Can you work these out from the model? Positions are in its coordinate system, mm. A direction names the side the tool comes from. Coordinates: 2 decimals unless noted, no trailing zeros. Loops run counter-clockwise (first coordinate to the right, second up) from the corner with the lowest first, then second, coordinate; pieces in that order, holes last.
```python
from build123d import *

# Parameters (mm, degrees)
BOSS_EXTRUDE1_DEPTH     = 46
BOSS_EXTRUDE2_DEPTH     = 54
CUT_EXTRUDE1_DEPTH      = 133.4990566
CUT_EXTRUDE1_DEPTH_BACK = 133.4990566
CUT_EXTRUDE2_DEPTH      = 126.888839855
CUT_EXTRUDE2_DEPTH_BACK = 126.888839855
F_12_0MM_DOWEL_HOLE1_D  = 12
SKETCH14_W              = 28
SKETCH14_H              = 28
SKETCH14_R              = 6
CUT_EXTRUDE5_DEPTH      = 10
SKETCH15_R              = 4
CUT_EXTRUDE6_DEPTH      = 54
CUT_EXTRUDE7_DEPTH      = 21
CHAMFER2_SIZE           = 2
FILLET1_R               = 8
CHAMFER3_SIZE           = 1


with BuildPart() as part:
    # Sketch1 → Boss-Extrude1 (new body)
    with BuildSketch(Plane.XY):
        Polygon((-104, 0), (104, 0), (99.985564599, 14), (-99.985564599, 14), align=None)
    extrude(amount=BOSS_EXTRUDE1_DEPTH)

    # Sketch2 → Boss-Extrude2 (add)
    with BuildSketch(Plane(origin=(0, 14, 0), x_dir=(1, 0, 0), z_dir=(0, 1, 0))):
        with BuildLine():
            Line((-48.856934001, 0), (48.856934001, 0))
            ThreePointArc((48.856934001, 0), (54, -23), (48.856934001, -46))
            Line((48.856934001, -46), (-48.856934001, -46))
            ThreePointArc((-48.856934001, -46), (-54, -23), (-48.856934001, 0))
        make_face()
    extrude(amount=BOSS_EXTRUDE2_DEPTH)

    # Sketch3 → Cut-Extrude1 (cut, two sides: drawn at the far end of the back side and taken through both)
    with BuildSketch(Plane.XY.offset(46).offset(-CUT_EXTRUDE1_DEPTH_BACK)):
        with BuildLine():
            Line((28, 52), (28, 68))
            Line((28, 68), (-28, 68))
            Line((-28, 68), (-28, 52))
            Line((-28, 52), (-23.664319132, 52))
            ThreePointArc((-23.664319132, 52), (0, 24), (23.664319132, 52))
            Line((23.664319132, 52), (28, 52))
        make_face()
    extrude(amount=CUT_EXTRUDE1_DEPTH + CUT_EXTRUDE1_DEPTH_BACK, mode=Mode.SUBTRACT)

    # Sketch4 → Cut-Extrude2 (cut, two sides: drawn at the far end of the back side and taken through both)
    with BuildSketch(Plane(origin=(0, 14, 0), x_dir=(1, 0, 0), z_dir=(0, 1, 0)).offset(-CUT_EXTRUDE2_DEPTH_BACK)):
        with BuildLine():
            Line((77, -17), (85, -17))
            ThreePointArc((85, -17), (91, -23), (85, -29))
            Line((85, -29), (77, -29))
            ThreePointArc((77, -29), (71, -23), (77, -17))
        make_face()
        with BuildLine():
            Line((-77, -17), (-85, -17))
            ThreePointArc((-85, -17), (-91, -23), (-85, -29))
            Line((-85, -29), (-77, -29))
            ThreePointArc((-77, -29), (-71, -23), (-77, -17))
        make_face()
    extrude(amount=CUT_EXTRUDE2_DEPTH + CUT_EXTRUDE2_DEPTH_BACK, mode=Mode.SUBTRACT)

    # Ø12.0mm Dowel Hole1 (through all)
    with Locations(Plane(origin=(0, 68, 0), x_dir=(1, 0, 0), z_dir=(0, 1, 0))):
        with Locations((39, -23)):
            f_12_0mm_dowel_hole1 = Hole(F_12_0MM_DOWEL_HOLE1_D / 2)

    # Mirror1: Ø12.0mm Dowel Hole1 across plane
    add(f_12_0mm_dowel_hole1.mirror(Plane(origin=(0, 0, 0), x_dir=(0, 0, 1), z_dir=(1, 0, 0))), mode=Mode.SUBTRACT)

    # Sketch14 → Cut-Extrude5 (cut)
    # profile 1 of 2: a face of its own
    with BuildSketch(Plane.XZ):
        with Locations((-39, 23)):
            Rectangle(SKETCH14_W, SKETCH14_H)
        with Locations(Location((-39, 23, 0), (0, 0, 90))):
            Circle(SKETCH14_R, mode=Mode.SUBTRACT)
    # profile 2 of 2: a face of its own
    with BuildSketch(Plane.XZ):
        with Locations((39, 23)):
            Rectangle(SKETCH14_W, SKETCH14_H)
        with Locations(Location((39, 23, 0), (0, 0, 90))):
            Circle(SKETCH14_R, mode=Mode.SUBTRACT)
    extrude(amount=-CUT_EXTRUDE5_DEPTH, mode=Mode.SUBTRACT)

    # Sketch15 → Cut-Extrude6 (cut)
    with BuildSketch(Plane(origin=(0, 68, 0), x_dir=(1, 0, 0), z_dir=(0, 1, 0))):
        with Locations(Location((0, -23, 0), (0, 0, 180))):
            Circle(SKETCH15_R)
    extrude(amount=-CUT_EXTRUDE6_DEPTH, mode=Mode.SUBTRACT)

    # Sketch18 → Cut-Extrude7 (cut, symmetric)
    with BuildSketch(Plane.XY.offset(23)):
        Polygon((-97.5, 0), (-96.926509228, 2), (96.926509228, 2), (97.5, 0), align=None)
    extrude(amount=CUT_EXTRUDE7_DEPTH, both=True, mode=Mode.SUBTRACT)

    # Chamfer2
    chamfer2_edges = [part.edges().sort_by_distance(p)[0] for p in [
        (0, 24, 0),
        (0, 24, 46),
    ]]
    chamfer(chamfer2_edges, length=CHAMFER2_SIZE)

    # Fillet1
    fillet1_edges = [part.edges().sort_by_distance(p)[0] for p in [
        (54, 14, 23),
        (-54, 14, 23),
    ]]
    fillet(fillet1_edges, radius=FILLET1_R)

    # Chamfer3
    chamfer3_edges = [part.edges().sort_by_distance(p)[0] for p in [
        (-71, 14, 23),
        (-81, 14, 29),
        (-91, 14, 23),
        (-81, 14, 17),
        (81, 14, 17),
        (81, 14, 29),
        (91, 14, 23),
        (71, 14, 23),
    ]]
    chamfer(chamfer3_edges, length=CHAMFER3_SIZE)


solid = part.part
```
(1) I want a section at D-D on x = -38. Write out the boundary of the cut face in (y, z), then the cut area to 3 significant figures.
Check values:
outline: (0, 0) - (68, 0) - (68, 17.08) - (10, 17.08) - (10, 9) - (2, 9) - (2, 2) - (0, 2) - close; (0, 44) - (2, 44) - (2, 37) - (10, 37) - (10, 28.92) - (68, 28.92) - (68, 46) - (0, 46) - close
area: 2,130 mm2
(2) I want a section at B-B on x = 39. Write out the boundary of the cut face in (y, z).
Check values:
outline: (0, 0) - (68, 0) - (68, 17) - (10, 17) - (10, 9) - (2, 9) - (2, 2) - (0, 2) - close; (0, 44) - (2, 44) - (2, 37) - (10, 37) - (10, 29) - (68, 29) - (68, 46) - (0, 46) - close
(3) Which directions (+Z, -Z, +X, -X, +Y, -Y) give clear straight access to the entire face, cutting with the end or side of a thin tool? Please do faces 3 (the conical face through (-70.8, 13.2, 22.9)), 4 (the flat face through (-28, 60, 23)), 5 (the cylindrical face through (91, 7, 23)), 6 (the flat face through (-53, 6, 23)).
Check values:
face 3: +Y
face 4: +Z, -Z, +Y
face 5: +Y, -Y
face 6: -Y
(4) I want a section at A-A on y = 58. Write out the boundary of the cut face in (x, z).
Check values:
outline: (-48.86, 0) - (-28, 0) - (-28, 46) - (-48.86, 46) arc R54 ccw to start; (28, 0) - (48.86, 0) arc R54 ccw to (48.86, 46) - (28, 46) - close; hole circle Ø12 at (-39, 23); hole circle Ø12 at (39, 23)
(5) If I drill on probe 1 along X at (y, z) = (22.25, 23); probe 2 along Z at (x, y) = (0, 18); probe 3 along X at (y, z) = (33, 19.5) (3 decimals), over which ranges is the centre line in solid material (lowest first)?
Check values:
probe 1: x = -54 to -45, -33 to -4, 4 to 33, 45 to 54
probe 2: z = 0 to 19, 27 to 46
probe 3: x = -53.886 to -43.873, -34.127 to -18.735, 18.735 to 34.127, 43.873 to 53.886
(6) If we mould it in two halves opening along X, with no side actions, what happens to faces 1 (the flat face through (-78, 14, 12)), 2 (the flat face through (-39, 6, 37))? For each: released by +X, released by -X, zero draft, split by the parting line, or undercut.
Check values:
face 1: zero draft
face 2: undercut
(7) I want a section at C-C on y = 48. Write out the boundary of the cut face in (x, z), then the cut area to 3 significant figures.
Check values:
outline: (-48.86, 0) - (-26, 0) - (-24, 2) - (-24, 44) - (-26, 46) - (-48.86, 46) arc R54 ccw to start; (24, 2) - (26, 0) - (48.86, 0) arc R54 ccw to (48.86, 46) - (26, 46) - (24, 44) - close; hole circle Ø12 at (-39, 23); hole circle Ø12 at (39, 23)
area: 2,370 mm2
(8) I'm going to push flat-ended pins straight in: pin 1 (12 mm diameter, centred on x = -3.5, z = 14.5, fed in from +Y); pin 2 (1.3 mm diameter, centred on x = 25, z = 19.5, fed in from +Y); pin 3 (6 mm diameter, centred on y = 59, z = 8, fed in from -X). Where does each tip first touch, or does it pass through?
Check values:
pin 1: stops at y = 25.96
pin 2: stops at y = 52
pin 3: stops at x = -52.65
